```python
from build123d import *

# Parameters (mm, degrees)
SKETCH1_R           = 2.5527
SKETCH1_R_2         = 3.048
SKETCH1_R_3         = 14.351
BOSS_EXTRUDE1_DEPTH = 6.35


with BuildPart() as part:
    # Sketch1 → Boss-Extrude1 (new body)
    with BuildSketch(Plane.XY):
        Polygon((0, -9.525), (-139.7, -9.525), (-139.7, 152.4), (139.7, 152.4), (139.7, -9.525), align=None)
        Circle(SKETCH1_R, mode=Mode.SUBTRACT)
        with Locations((12.7, 0)):
            Circle(SKETCH1_R, mode=Mode.SUBTRACT)
        with Locations((25.4, 0)):
            Circle(SKETCH1_R, mode=Mode.SUBTRACT)
        with Locations((38.1, 0)):
            Circle(SKETCH1_R, mode=Mode.SUBTRACT)
        with Locations((50.8, 0)):
            Circle(SKETCH1_R, mode=Mode.SUBTRACT)
        with Locations(Location((-50.8, 0, 0), (0, 0, 180))):
            Circle(SKETCH1_R, mode=Mode.SUBTRACT)
        with Locations(Location((-38.1, 0, 0), (0, 0, 180))):
            Circle(SKETCH1_R, mode=Mode.SUBTRACT)
        with Locations(Location((-25.4, 0, 0), (0, 0, 180))):
            Circle(SKETCH1_R, mode=Mode.SUBTRACT)
        with Locations(Location((-12.7, 0, 0), (0, 0, 180))):
            Circle(SKETCH1_R, mode=Mode.SUBTRACT)
        with Locations((-82.55, 22.225)):
            Circle(SKETCH1_R, mode=Mode.SUBTRACT)
        with Locations((-85.952954744, 9.525)):
            Circle(SKETCH1_R, mode=Mode.SUBTRACT)
        with Locations((-95.25, 0.227954744)):
            Circle(SKETCH1_R, mode=Mode.SUBTRACT)
        with Locations((-107.95, -3.175)):
            Circle(SKETCH1_R, mode=Mode.SUBTRACT)
        with Locations((-120.65, 0.227954744)):
            Circle(SKETCH1_R, mode=Mode.SUBTRACT)
        with Locations((-129.947045256, 9.525)):
            Circle(SKETCH1_R, mode=Mode.SUBTRACT)
        with Locations((-133.35, 22.225)):
            Circle(SKETCH1_R, mode=Mode.SUBTRACT)
        with Locations((-129.947045256, 34.925)):
            Circle(SKETCH1_R, mode=Mode.SUBTRACT)
        with Locations((-120.65, 44.222045256)):
            Circle(SKETCH1_R, mode=Mode.SUBTRACT)
        with Locations((-107.95, 47.625)):
            Circle(SKETCH1_R, mode=Mode.SUBTRACT)
        with Locations((-95.25, 44.222045256)):
            Circle(SKETCH1_R, mode=Mode.SUBTRACT)
        with Locations((-85.952954744, 34.925)):
            Circle(SKETCH1_R, mode=Mode.SUBTRACT)
        with Locations((100.542736572, 141.867296719)):
            Circle(SKETCH1_R_2, mode=Mode.SUBTRACT)
        with Locations((104.775, 101.6)):
            Circle(SKETCH1_R_2, mode=Mode.SUBTRACT)
        with Locations((100.542736572, 61.332703281)):
            Circle(SKETCH1_R_2, mode=Mode.SUBTRACT)
        with Locations((88.030916509, 22.825280652)):
            Circle(SKETCH1_R_2, mode=Mode.SUBTRACT)
        with Locations((-107.95, 22.225)):
            Circle(SKETCH1_R_3, mode=Mode.SUBTRACT)
        with Locations((-88.9, 101.6)):
            Circle(SKETCH1_R_3, mode=Mode.SUBTRACT)
        with Locations((-56.893674009, 28.423794002)):
            Circle(SKETCH1_R_3, mode=Mode.SUBTRACT)
    extrude(amount=BOSS_EXTRUDE1_DEPTH)


solid = part.part
```
Could you check a few things on this model? Use its own coordinates, in mm. Coordinates: 2 decimals unless noted, no trailing zeros. Return JSON: item names as keys, results as strings.
(1) I need wall thicknesses on L1, parallel to X at y = 101, z = 4.5; L2, parallel to Y at x = -110, z = 4.75 (3 decimals); L3, parallel to Y at x = 0, z = 3.75 (3 decimals). Which ranges of each line are inside material? Lowest first, please.
Numbers:
{"L1": "x = -139.7 to -103.24, -74.56 to 101.79, 107.76 to 139.7", "L2": "y = -9.525 to -4.696, -1.654 to 8.021, 36.429 to 46.104, 49.146 to 152.4", "L3": "y = -9.525 to -2.553, 2.553 to 152.4"}
(2) We'd pull the mould along Y, two halves only. Please class faces 1 (the flat face through (139.7, 73, 3)), 2 (the cylindrical face through (-127.59, 8.55, 3.13)), 3 (the flat face through (-2, 152.4, 3)): +Y half, -Y half, draft (parallel to the pull), parting line (faces both ways), or undercut.
Numbers:
{"face 1": "draft", "face 2": "undercut", "face 3": "+Y half"}
(3) I'm going to push a flat-ended pin straight in: pin 1 (4.5 mm diameter, centred on x = -82.55, y = 22.225, fed in from +Z). Where does the tip first touch, or does it pass through?
Numbers:
{"pin 1": "passes through"}
(4) Imagine slicing it at A-A, the plane z = 4.75. Count the separate pieces of the cut face and the enclosed holes in it, then the cut area to 3 significant figures.
Numbers:
{"separate pieces": "1", "enclosed holes": "28", "area": "42,800 mm2"}
